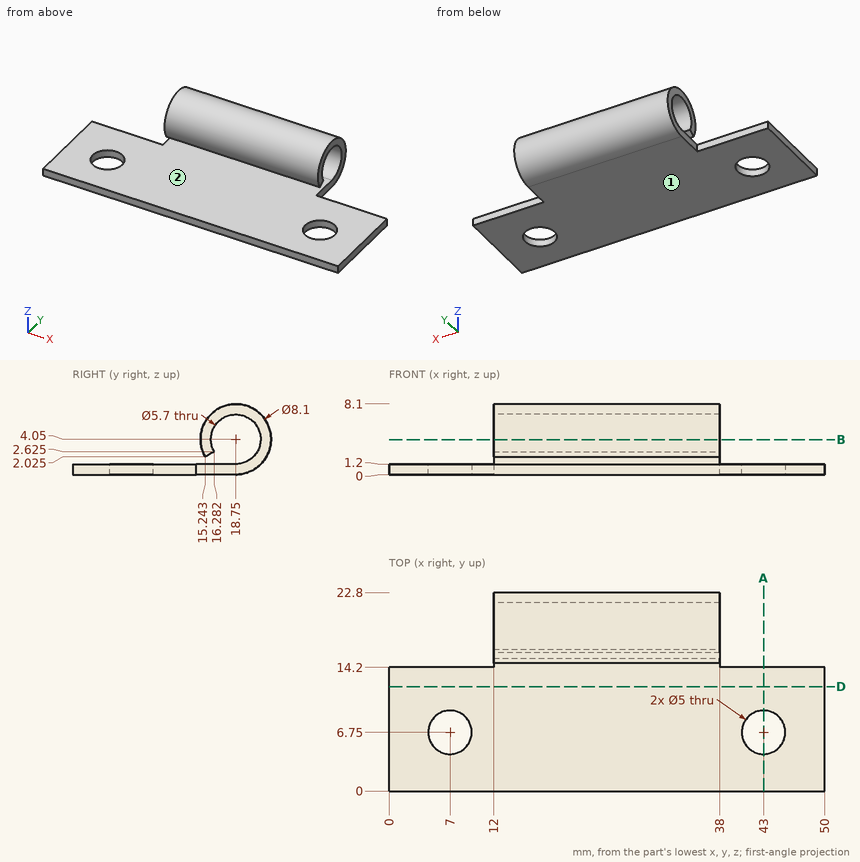
Study the drawing (mm; zero at the part's minimum x, y, z) and answer. Give positions to 0.01 mm unless a question says otherwise; leave off trailing zeros. Write each loop counter-clockwise with the first axis right and the second up, starting at its lowest first coordinate (ties: lowest second). Pieces come first, ordered by that corner, then holes.
(1) The mould has two halves that part along Z. Classify the marked faces 1 and 2: pulls with the +Z half, pulls with the -Z half, needs draft (parallel to the pull), parting line crosses it, or undercut.
Final values:
face 1: pulls with the -Z half
face 2: undercut
(2) The part is cut by section A-A on x = 43. Write down the section's boundary in (y, z).
Final values:
outline: (0, 0) - (4.25, 0) - (4.25, 1.2) - (0, 1.2) - close; (9.25, 0) - (14.2, 0) - (14.2, 1.2) - (9.25, 1.2) - close
(3) The part is cut by section D-D on y = 12. Write down the section's boundary in (x, z).
Final values:
outline: (0, 0) - (50, 0) - (50, 1.2) - (0, 1.2) - close
(4) Straight lines are drawn through the part: line 1 (Y direction, x = 30.75, z = 4.05); line 2 (Y direction, x = 7, z = 0.75); line 3 (Z direction, x = 38, y = 9.5). For each, find the intervals that lie inside material, in ascending order.
Final values:
line 1: y = 14.7 to 15.9, 21.6 to 22.8
line 2: y = 0 to 4.25, 9.25 to 14.2
line 3: z = 0 to 1.2
(5) Flat-ended cylindrical pins translate along their axes: pin 1 Ø1.5 at (x, z) = (18.5, 1) entering from +Y; pin 2 Ø2 at (x, y) = (40, 4) entering from +Z; pin 3 Ø4 at (y, z) = (16.5, 6) entering from -X. Find the tip coordinate at first contact, or state that the pin passes through.
Final values:
pin 1: stops at y = 22.08
pin 2: stops at z = 1.2
pin 3: stops at x = 12
(6) The part is cut by section B-B on z = 4. Write down the section's boundary in (x, y).
Final values:
outline: (12, 14.7) - (38, 14.7) - (38, 15.9) - (12, 15.9) - close; (12, 21.6) - (38, 21.6) - (38, 22.8) - (12, 22.8) - close
